Design review of the part built by this model. Coordinates are the model's own, in mm. Face numbers are marked on the shaded views. A direction names the side the tool comes from. Give positions to 0.01 mm unless a question says otherwise; leave off trailing zeros. Order: outer loops, then holes, each group sorted by start corner. A loop starts at its lowest first (then second) coordinate and runs counter-clockwise, first axis right, second up. Notation, with made-up numbers: (-13.75, 77.25) -> (30.25, 77.25) arc R22 cw to (30.25, 86.25) -> close; hole circle Ø7 at (46.5, -1). An arc over 180 degrees is marked (long way). Answer in a Markdown table with one row per item. Add a question column.
```python
from build123d import *
from build123d.topology import SkipClean

# Parameters (mm, degrees)
BOSS_EXTRUDE1_DEPTH  = 20
SKETCH2_W            = 100
SKETCH2_H            = 20
CUT_EXTRUDE1_DEPTH   = 20
FILLET1_R            = 9.75
FILLET1_OF_MIRROR4_R = 9.75
SKETCH4_R            = 2.1
CUT_EXTRUDE3_DEPTH   = 20


with BuildPart() as part:
    # Sketch1 → Boss-Extrude1 (new body)
    with BuildSketch(Plane(origin=(0, 0, 0), x_dir=(1, 0, 0), z_dir=(0, 1, 0))):
        with BuildLine():
            Line((22.360679775, 20), (130, 20))
            Line((130, 20), (130, -20))
            Line((130, -20), (22.360679775, -20))
            ThreePointArc((22.360679775, -20), (12.247448714, -27.386127875), (0, -30))
            Line((0, -30), (0, -20))
            Line((0, -20), (0, 20))
            Line((0, 20), (0, 30))
            ThreePointArc((0, 30), (12.247448714, 27.386127875), (22.360679775, 20))
        make_face()
    boss_extrude1 = extrude(amount=BOSS_EXTRUDE1_DEPTH)

    # Sketch2 → Cut-Extrude1 (cut)
    with BuildSketch(Plane(origin=(0, 20, 0), x_dir=(1, 0, 0), z_dir=(0, 1, 0))):
        with BuildLine():
            Line((0, 17), (0, -17))
            ThreePointArc((0, -17), (17, 0), (0, 17))
        make_face()
        with Locations((80, 0)):
            Rectangle(SKETCH2_W, SKETCH2_H)
    cut_extrude1 = extrude(amount=-CUT_EXTRUDE1_DEPTH, mode=Mode.SUBTRACT)

    # Fillet1
    fillet1_edges = [part.edges().sort_by_distance(p)[0] for p in [
        (130, 10, -20),
        (130, 10, 20),
    ]]
    fillet(fillet1_edges, radius=FILLET1_R)

    # Mirror4: Boss-Extrude1, Cut-Extrude1 across plane
    with SkipClean():  # the faces are left unmerged after this step: merging them gives an invalid solid
        add(boss_extrude1.mirror(Plane(origin=(0, 0, 0), x_dir=(0, 0, 1), z_dir=(1, 0, 0))))
        add(cut_extrude1.mirror(Plane(origin=(0, 0, 0), x_dir=(0, 0, 1), z_dir=(1, 0, 0))), mode=Mode.SUBTRACT)
    add(part.part.scale(1), mode=Mode.REPLACE)  # the faces are merged on a copy

    # Fillet1 of Mirror4
    fillet1_of_mirror4_edges = [part.edges().sort_by_distance(p)[0] for p in [
        (-130, 10, -20),
        (-130, 10, 20),
    ]]
    fillet(fillet1_of_mirror4_edges, radius=FILLET1_OF_MIRROR4_R)

    # Sketch4 → Cut-Extrude3 (cut)
    with BuildSketch(Plane(origin=(0, 20, 0), x_dir=(1, 0, 0), z_dir=(0, 1, 0))):
        with Locations(Location((21, 0, 0), (0, 0, 270))):
            Circle(SKETCH4_R)
        with Locations(Location((14.849242405, -14.849242405, 0), (0, 0, 270))):
            Circle(SKETCH4_R)
        with Locations(Location((0, -21, 0), (0, 0, 270))):
            Circle(SKETCH4_R)
        with Locations(Location((-14.849242405, -14.849242405, 0), (0, 0, 270))):
            Circle(SKETCH4_R)
        with Locations(Location((-21, 0, 0), (0, 0, 270))):
            Circle(SKETCH4_R)
        with Locations(Location((-14.849242405, 14.849242405, 0), (0, 0, 270))):
            Circle(SKETCH4_R)
        with Locations(Location((0, 21, 0), (0, 0, 270))):
            Circle(SKETCH4_R)
        with Locations(Location((14.849242405, 14.849242405, 0), (0, 0, 270))):
            Circle(SKETCH4_R)
    extrude(amount=-CUT_EXTRUDE3_DEPTH, mode=Mode.SUBTRACT)


solid = part.part
```
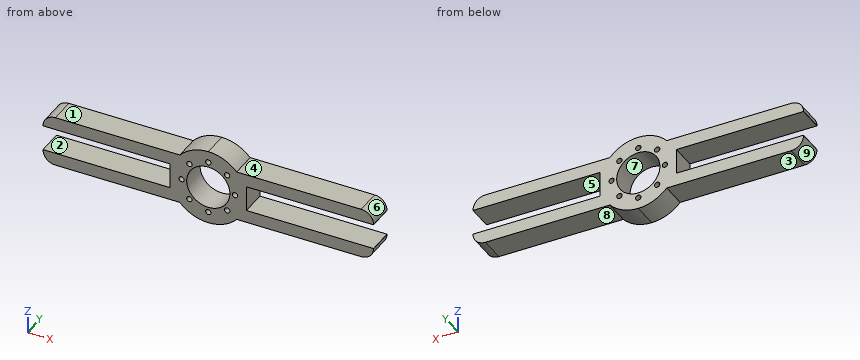
1) Add section C-C, the plane z = 7.5. Write out the cut boundary in (x, y).
2) Machinability: for the marked faces 1, 2, 3, 4 and 5, which of the approach directions +Z, -Z, +X, -X, +Y, -Y give a long, thin tool a straight path to every point of the face, cutting with its end or side? Answer none if there is none.
3) Add section B-B, the plane y = 6. Give the number of separate pieces and of enclosed holes in the cut face, and give its area (3 significant figures).
4) Mouldability with a two-part tool opening along X and no side actions: class the marked faces 6, 7, 8 and 9 as +X half, -X half, draft (parallel to the pull), parting line (faces both ways), or undercut.
5) Add section A-A, the plane x = -87. Write out the cut boundary in (y, z).
6) Clearance check with flat-ended pins moving along their axes: P1, Ø5, axis at x = 14.85, z = -14.85, coming from the -Y side; P2, Ø6, axis at x = -98, y = 14, coming from the -Z side; P3, Ø12, axis at x = 14, y = 4, coming from the -Z side; P4, Ø6, axis at y = 9.5, z = 5, coming from the -X side. State where each tip first meets the part, or that it passes through.
7) For L1, parallel to X at y = 13, z = 0; L2, parallel to Z at x = -91.5, y = 16; L3, parallel to X at y = 14, z = -14, list the stretches that pass through material, from the lowest coordinate up.
Verdict:
| question | item | result |
|---|---|---|
| 1 | outline | (-30, 0) -> (-15.26, 0) -> (-15.26, 20) -> (-30, 20) -> close; (15.26, 0) -> (30, 0) -> (30, 20) -> (15.26, 20) -> close |
| 2 | face 1 | +Z, -X, +Y, -Y |
| 2 | face 2 | -X, +Y, -Y |
| 2 | face 3 | -Z, -X, +Y, -Y |
| 2 | face 4 | +Z, +X, +Y, -Y |
| 2 | face 5 | +X, +Y, -Y |
| 3 | separate pieces | 1 |
| 3 | enclosed holes | 9 |
| 3 | area | 5,920 mm2 |
| 4 | face 6 | +X half |
| 4 | face 7 | undercut |
| 4 | face 8 | draft |
| 4 | face 9 | -X half |
| 5 | outline | (0, -20) -> (20, -20) -> (20, -10) -> (0, -10) -> close; (0, 10) -> (20, 10) -> (20, 20) -> (0, 20) -> close |
| 6 | P1 | stops at y = 0 |
| 6 | P2 | stops at z = -20 |
| 6 | P3 | stops at z = -28.91 |
| 6 | P4 | stops at x = -30 |
| 7 | L1 | x = -30 to -23.1, -18.9 to -17, 17 to 18.9, 23.1 to 30 |
| 7 | L2 | z = -20 to -10, 10 to 20 |
| 7 | L3 | x = -129.25 to -16.77, -12.93 to -9.64, 9.64 to 12.93, 16.77 to 129.25 |
